Check sheet for the modelled part. Datum: model origin and axes. Units: mm. Coordinates: 2 decimals unless noted, no trailing zeros. Loops run counter-clockwise (first coordinate to the right, second up) from the corner with the lowest first, then second, coordinate; pieces in that order, holes last. Notation, with made-up numbers: (40.25, 8.5) -> (44.25, 8.5) arc R19 ccw to (44.25, 30.5) -> close; hole circle Ø7 at (87.5, -9.5). An arc over 180 degrees is marked (long way). Use CSV: the item, a comma, the result in double quotes. Start each with the question number.
1. Sectioned sample at B-B, the plane z = 1.35. Record the cut outline in (x, y).
2. Thickness scan on L1, parallel to X at y = 0.75, z = 1.65; L2, parallel to X at y = 7, z = -1.4; L3, parallel to Z at x = -4, y = 3. Record the ranges inside material, lowest first.
3. Gauge pin test, flat end, axial feed: pin 1 (2 mm diameter, centred on y = 4, z = -1.5, fed in from +X). Record the tip position at first contact, or that the pin passes through.
4. Sectioned sample at A-A, the plane y = 3. Record the cut outline in (x, z), and give its area (3 significant figures).
```python
from build123d import *

# Parameters (mm, degrees)
SKETCH1_R           = 4.5
BOSS_EXTRUDE1_DEPTH = 7.9371
SKETCH2_W           = 9.255904856
SKETCH2_H           = 5.023128632
CUT_EXTRUDE1_DEPTH  = 7.9371
SKETCH3_W           = 9.61068527
SKETCH3_H           = 3.540778784
CUT_EXTRUDE2_DEPTH  = 7.9371


with BuildPart() as part:
    # Sketch1 → Boss-Extrude1 (new body)
    with BuildSketch(Plane(origin=(0, 0, 0), x_dir=(1, 0, 0), z_dir=(0, 1, 0))):
        Circle(SKETCH1_R)
    extrude(amount=BOSS_EXTRUDE1_DEPTH)

    # Sketch2 → Cut-Extrude1 (cut)
    with BuildSketch(Plane(origin=(0, 7.9371, 0), x_dir=(1, 0, 0), z_dir=(0, 1, 0))):
        with Locations((-0.035126774, 4.926530004)):
            Rectangle(SKETCH2_W, SKETCH2_H)
    extrude(amount=-CUT_EXTRUDE1_DEPTH, mode=Mode.SUBTRACT)

    # Sketch3 → Cut-Extrude2 (cut)
    with BuildSketch(Plane(origin=(0, 7.9371, 0), x_dir=(1, 0, 0), z_dir=(0, 1, 0))):
        with Locations((0.263450802, -3.750791404)):
            Rectangle(SKETCH3_W, SKETCH3_H)
    extrude(amount=-CUT_EXTRUDE2_DEPTH, mode=Mode.SUBTRACT)


solid = part.part
```
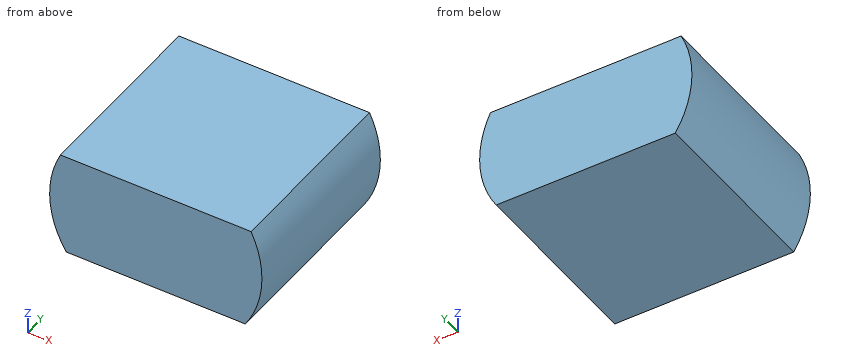
Completed:
1,outline,"(-4.29, 0) -> (4.29, 0) -> (4.29, 7.94) -> (-4.29, 7.94) -> close"
2,L1,"-4.19 to 4.19"
2,L2,"-4.28 to 4.28"
2,L3,"-2.06 to 1.98"
3,pin 1,"x = 4.47"
4,outline,"(-4.04, 1.98) arc R4.5 ccw to (-3.8, -2.41) -> (3.8, -2.41) arc R4.5 ccw to (4.04, 1.98) -> close"
4,area,"37.9 mm²"
